Can you work these out from the model? Positions are in its coordinate system, mm. A direction names the side the tool comes from. Round coordinates to 2 decimals unless told otherwise and drop trailing zeros. Loops run counter-clockwise (first coordinate to the right, second up) from the corner with the lowest first, then second, coordinate; pieces in that order, holes last. Notation, with made-up numbers: (-37, 78.5) - (-1, 78.5) arc R16 ccw to (-1, 103.5) - close; hole circle Ø9 at (79.5, 44). An arc over 180 degrees is marked (long way). Answer as CSV lines item,"result".
```python
from build123d import *

# Parameters (mm, degrees)
SKETCH1_W           = 22.5552
SKETCH1_H           = 12.7
BOSS_EXTRUDE1_DEPTH = 1
SKETCH2_W           = 5
SKETCH2_H           = 7.3
CUT_EXTRUDE1_DEPTH  = 1
SKETCH3_W           = 5
SKETCH3_H           = 5
CUT_EXTRUDE2_DEPTH  = 1
BOSS_EXTRUDE2_DEPTH = 1
SKETCH5_W           = 26.5552
SKETCH5_H           = 16.7
BOSS_EXTRUDE3_DEPTH = 1
CUT_EXTRUDE3_DEPTH  = 1
CUT_EXTRUDE4_DEPTH  = 1
CUT_EXTRUDE5_START  = -4
CUT_EXTRUDE5_DEPTH  = 5
SKETCH10_W          = 22.5552
SKETCH10_H          = 2
BOSS_EXTRUDE4_DEPTH = 2
SKETCH11_W          = 8.919893548
SKETCH11_H          = 0.730490532
CUT_EXTRUDE6_DEPTH  = 3
SKETCH12_W          = 22.5552
SKETCH12_H          = 1.5
BOSS_EXTRUDE5_DEPTH = 2
SKETCH13_W          = 3
SKETCH13_H          = 1.5
CUT_EXTRUDE7_DEPTH  = 2
SKETCH14_W          = 2.125
SKETCH14_H          = 1.226869322
CUT_EXTRUDE8_DEPTH  = 1


with BuildPart() as part:
    # Sketch1 → Boss-Extrude1 (new body)
    with BuildSketch(Plane(origin=(0, 0, 0), x_dir=(1, 0, 0), z_dir=(0, 1, 0))):
        with Locations((-28.763088774, 14.606547542)):
            Rectangle(SKETCH1_W, SKETCH1_H)
    extrude(amount=BOSS_EXTRUDE1_DEPTH)

    # Sketch2 → Cut-Extrude1 (cut)
    with BuildSketch(Plane(origin=(0, 1, 0), x_dir=(1, 0, 0), z_dir=(0, 1, 0))):
        with Locations((-37.540688774, 14.606547542)):
            Rectangle(SKETCH2_W, SKETCH2_H)
    extrude(amount=-CUT_EXTRUDE1_DEPTH, mode=Mode.SUBTRACT)

    # Sketch3 → Cut-Extrude2 (cut)
    with BuildSketch(Plane(origin=(0, 1, 0), x_dir=(1, 0, 0), z_dir=(0, 1, 0))):
        with Locations((-19.985488774, 13.756547542)):
            Rectangle(SKETCH3_W, SKETCH3_H)
    extrude(amount=-CUT_EXTRUDE2_DEPTH, mode=Mode.SUBTRACT)

    # Sketch4 → Boss-Extrude2 (add)
    with BuildSketch(Plane.XZ):
        Polygon((-40.040688774, -8.256547542), (-40.040688774, -8.756547542), (-17.985488774, -8.756547542), (-17.985488774, -10.256547542), (-17.485488774, -10.256547542), (-17.485488774, -8.256547542), align=None)
        Polygon((-17.985488774, -20.456547542), (-40.040688774, -20.456547542), (-40.040688774, -20.956547542), (-17.485488774, -20.956547542), (-17.485488774, -18.456547542), (-17.985488774, -18.456547542), align=None)
    extrude(amount=BOSS_EXTRUDE2_DEPTH)

    # Sketch5 → Boss-Extrude3 (add)
    with BuildSketch(Plane(origin=(0, 1, 0), x_dir=(1, 0, 0), z_dir=(0, 1, 0))):
        with Locations((-26.763088774, 14.606547542)):
            Rectangle(SKETCH5_W, SKETCH5_H)
    extrude(amount=BOSS_EXTRUDE3_DEPTH)

    # Sketch6 → Cut-Extrude3 (cut)
    with BuildSketch(Plane(origin=(0, 2, 0), x_dir=(1, 0, 0), z_dir=(0, 1, 0))):
        Polygon((-40.040688774, 13.37967822), (-37.915688774, 12.152808898), (-35.790688774, 13.37967822), (-35.790688774, 15.833416864), (-37.915688774, 17.060286186), (-40.040688774, 15.833416864), align=None)
    extrude(amount=-CUT_EXTRUDE3_DEPTH, mode=Mode.SUBTRACT)

    # Sketch7 → Cut-Extrude4 (cut)
    with BuildSketch(Plane(origin=(0, 1, 0), x_dir=(-1, 0, 0), z_dir=(0, -1, 0))):
        Polygon((17.735488774, 14.983416864), (15.610488774, 16.210286186), (13.485488774, 14.983416864), (13.485488774, 12.52967822), (15.610488774, 11.302808898), (17.735488774, 12.52967822), align=None)
    extrude(amount=-CUT_EXTRUDE4_DEPTH, mode=Mode.SUBTRACT)

    # Sketch8 → Cut-Extrude5 (cut)
    with BuildSketch(Plane(origin=(0, 2, 0), x_dir=(1, 0, 0), z_dir=(0, 1, 0)).offset(CUT_EXTRUDE5_START)):
        with BuildLine():
            Line((-13.485488774, 22.956547542), (-22.127760886, 22.956547542))
            add(Edge.make_bspline(
                [(-22.127760886, 22.956547542), (-17.367981555, 22.956547542), (-14.30272025, 21.87197064), (-13.485488774, 18.176213027)],
                knots=[0, 0, 0, 0, 1, 1, 1, 1], degree=3))
            Line((-13.485488774, 18.176213027), (-13.485488774, 22.956547542))
        make_face()
    cut_extrude5 = extrude(amount=CUT_EXTRUDE5_DEPTH, mode=Mode.SUBTRACT)

    # Mirror2: Cut-Extrude5 across plane
    add(cut_extrude5.mirror(Plane.XY.offset(-14.61)), mode=Mode.SUBTRACT)

    # Sketch10 → Boss-Extrude4 (add)
    with BuildSketch(Plane(origin=(0, 1, 0), x_dir=(-1, 0, 0), z_dir=(0, -1, 0))):
        with Locations((28.763088774, 7.256547542)):
            Rectangle(SKETCH10_W, SKETCH10_H)
        with Locations((28.763088774, 21.956547542)):
            Rectangle(SKETCH10_W, SKETCH10_H)
    extrude(amount=BOSS_EXTRUDE4_DEPTH)

    # Sketch11 → Cut-Extrude6 (cut)
    with BuildSketch(Plane(origin=(0, 2, 0), x_dir=(1, 0, 0), z_dir=(0, 1, 0))):
        with Locations((-17.667814112, 5.898207192)):
            Rectangle(SKETCH11_W, SKETCH11_H)
    extrude(amount=-CUT_EXTRUDE6_DEPTH, mode=Mode.SUBTRACT)

    # Sketch12 → Boss-Extrude5 (add)
    with BuildSketch(Plane(origin=(0, -1, 0), x_dir=(-1, 0, 0), z_dir=(0, -1, 0))):
        with Locations((28.763088774, 7.006547542)):
            Rectangle(SKETCH12_W, SKETCH12_H)
        with Locations((28.763088774, 22.206547542)):
            Rectangle(SKETCH12_W, SKETCH12_H)
    extrude(amount=BOSS_EXTRUDE5_DEPTH)

    # Sketch13 → Cut-Extrude7 (cut)
    with BuildSketch(Plane(origin=(0, -3, 0), x_dir=(-1, 0, 0), z_dir=(0, -1, 0))):
        with Locations((35.040688774, 7.006547542)):
            Rectangle(SKETCH13_W, SKETCH13_H)
        with Locations((35.040688774, 22.206547542)):
            Rectangle(SKETCH13_W, SKETCH13_H)
        with Locations((22.040688774, 7.006547542)):
            Rectangle(SKETCH13_W, SKETCH13_H)
        with Locations((22.040688774, 22.206547542)):
            Rectangle(SKETCH13_W, SKETCH13_H)
    extrude(amount=-CUT_EXTRUDE7_DEPTH, mode=Mode.SUBTRACT)

    # Sketch14 → Cut-Extrude8 (cut)
    with BuildSketch(Plane(origin=(0, 2, 0), x_dir=(1, 0, 0), z_dir=(0, 1, 0))):
        with Locations((-14.547988774, 15.596851525)):
            Rectangle(SKETCH14_W, SKETCH14_H)
        with Locations((-14.547988774, 11.916243559)):
            Rectangle(SKETCH14_W, SKETCH14_H)
    extrude(amount=-CUT_EXTRUDE8_DEPTH, mode=Mode.SUBTRACT)


solid = part.part
```
Q1. Imagine slicing it at D-D (x = -37). Write out the boundary of the cut face in (y, z), then the cut area to 3 significant figures.
Checks:
outline,"(-3, -22.96) - (2, -22.96) - (2, -16.53) - (1, -16.53) - (1, -18.26) - (0, -18.26) - (0, -20.46) - (-1, -20.46) - (-1, -21.46) - (-3, -21.46) - close; (-3, -7.76) - (-1, -7.76) - (-1, -8.76) - (0, -8.76) - (0, -10.96) - (1, -10.96) - (1, -12.68) - (2, -12.68) - (2, -6.26) - (-3, -6.26) - close"
area,"33.2 mm²"
Q2. We'd pull the mould along X, two halves only. Please class faces 1 (the flat face through (-13.485, 1.5, -17.2)), 2 (the flat face through (-29, -1, -21)), 3 (the flat face through (-29.2, -0.5, -8.757)), 4 (the flat face through (-33.541, -2, -22)): pulls with the +X half, pulls with the -X half, needs draft (parallel to the pull), parting line crosses it, or undercut.
Checks:
face 1,"pulls with the +X half"
face 2,"undercut"
face 3,"needs draft"
face 4,"undercut"
Q3. Imagine slicing it at A-A (y = -1.6). Write out the boundary of the cut face in (x, z).
Checks:
outline,"(-40.04, -22.96) - (-36.54, -22.96) - (-36.54, -21.46) - (-40.04, -21.46) - close; (-40.04, -7.76) - (-36.54, -7.76) - (-36.54, -6.26) - (-40.04, -6.26) - close; (-33.54, -22.96) - (-23.54, -22.96) - (-23.54, -21.46) - (-33.54, -21.46) - close; (-33.54, -7.76) - (-23.54, -7.76) - (-23.54, -6.26) - (-33.54, -6.26) - close; (-20.54, -22.96) - (-17.49, -22.96) - (-17.49, -21.46) - (-20.54, -21.46) - close; (-20.54, -7.76) - (-17.49, -7.76) - (-17.49, -6.26) - (-20.54, -6.26) - close"
Q4. Imagine slicing it at B-B (x = -33.25). Write out the boundary of the cut face in (y, z), then the cut area to 3 significant figures.
Checks:
outline,"(-3, -22.96) - (2, -22.96) - (2, -6.26) - (-3, -6.26) - (-3, -7.76) - (-1, -7.76) - (-1, -8.76) - (0, -8.76) - (0, -20.46) - (-1, -20.46) - (-1, -21.46) - (-3, -21.46) - close"
area,"44.4 mm²"
Q5. On a 3-axis mill with a long thin cutter (end or side, diameter ignored), from which of +Z, -Z, +X, -X, +Y, -Y can I reach the whole of each face in a straight line? I mean faces 5 (the flat face through (-19, -2, -7.757)), 6 (the flat face through (-36.541, -2, -7)), 7 (the flat face through (-16.66, 1.49, -11.91)), 8 (the flat face through (-17.485, 0, -20)), 9 (the flat face through (-36.868, 1.507, -12.758)). Say none if no direction works.
Checks:
face 5,"+X, -X, -Y"
face 6,"+Z, -Z, -Y"
face 7,"+X, +Y, -Y"
face 8,"+Z, -Z, +X, -Y"
face 9,"+Y, -Y"
Q6. I'm going to push flat-ended pins straight in: pin 1 Ø0.5 at (y, z) = (0.5, -14.5) entering from -X; pin 2 Ø0.8 at (y, z) = (-0.5, -9.5) entering from -X; pin 3 Ø1 at (x, y) = (-20, 0.5) entering from +Z. Where does each tip first touch, or does it pass through?
Checks:
pin 1,"x = -35.04"
pin 2,"x = -17.99"
pin 3,"z = -6.26"
Q7. If I drill on line 1 along Z through (x, y) = (-34.5, -0.6); line 2 along Z through (x, y) = (-29.5, -1.05); line 3 along Y through (x, z) = (-34, -9.25), over which ranges is the centre line in solid material (lowest first)? Write a range as [from, to].
Checks:
line 1,"[-22.96, -20.46], [-8.76, -6.26]"
line 2,"[-22.96, -21.46], [-7.76, -6.26]"
line 3,"[0, 2]"
